Can you work these out from the model? Positions are in its coordinate system, mm. Face numbers are marked on the shaded views. A direction names the side the tool comes from. Coordinates: 2 decimals unless noted, no trailing zeros. Loops run counter-clockwise (first coordinate to the right, second up) from the corner with the lowest first, then second, coordinate; pieces in that order, holes last. Notation, with made-up numbers: (-36, 31) -> (18, 31) arc R7 ccw to (18, 35) -> close; hole circle Ø6 at (-19.5, 87). An arc over 180 degrees is marked (long way). Put each result on its own line as item: value. Start each with the question number.
Item 1: If we section it at A-A on x = 74: State how many separate pieces and enclosed holes the cut face has, plus the area to 3 significant figures.
Item 2: Will these pins go through, and if not, where does the flat tip stop? P1, Ø2.5, axis at y = 9, z = 7, coming from the +X side; P2, Ø2.5, axis at y = 40, z = 6.5, coming from the +X side; P3, Ø2, axis at y = 11.5, z = 1, coming from the -X side; P4, Ø1.5, axis at y = -5, z = 4.5, coming from the +X side.
Item 3: We'd pull the mould along Y, two halves only. Please class the marked faces 1, 2 and 3: pulls with the +Y half, pulls with the -Y half, needs draft (parallel to the pull), parting line crosses it, or undercut.
Item 4: Please list where these lines run through material, in increasing order: L1, parallel to Y at x = 74, z = 3.45; L2, parallel to Y at x = 74, z = 0.7; L3, parallel to X at y = -1, z = 3. Write a range as from..to.
Item 5: For the marked faces 4 and 5, which set-ups out of +Z, -Z, +X, -X, +Y, -Y let a thin tool reach every point of the face, with its end or its side?
Item 6: If we section it at C-C on x = 0: Please give me the cut outline in (y, z), plus the area to 3 significant figures.
```python
from build123d import *

# Parameters (mm, degrees)
SKETCH1_R           = 3.05
SKETCH1_R_2         = 1.55
BOSS_EXTRUDE1_DEPTH = 9
CUT_EXTRUDE1_DEPTH  = 5
CHAMFER2_SIZE       = 2.7
SKETCH3_W           = 38
SKETCH3_H           = 38
CUT_EXTRUDE2_DEPTH  = 96.66216598
FILLET1_R           = 4
CHAMFER3_SIZE       = 2
SKETCH4_R           = 3.35
CUT_EXTRUDE3_DEPTH  = 1
CHAMFER4_SIZE       = 1.8


with BuildPart() as part:
    # Sketch1 → Boss-Extrude1 (new body)
    with BuildSketch(Plane.XY):
        with BuildLine():
            Line((84, 45.5), (84, 24))
            Line((84, 24), (84, -14.5))
            Line((84, -14.5), (84, -26.5))
            Line((84, -26.5), (18, -26.5))
            Line((18, -26.5), (-9.05, -8.967177323))
            Line((-9.05, -8.967177323), (-9.05, 0))
            ThreePointArc((-9.05, 0), (-8.604128548, 2.805614358), (-7.310448193, 5.334777148))
            Line((-7.310448193, 5.334777148), (22, 45.5))
            Line((22, 45.5), (84, 45.5))
        make_face()
        with Locations((34, 35.5)):
            Circle(SKETCH1_R, mode=Mode.SUBTRACT)
        with Locations((54, 35.5)):
            Circle(SKETCH1_R, mode=Mode.SUBTRACT)
        with Locations((74, 35.5)):
            Circle(SKETCH1_R_2, mode=Mode.SUBTRACT)
        with Locations((74, -20.5)):
            Circle(SKETCH1_R_2, mode=Mode.SUBTRACT)
        with BuildLine():
            Line((43, 23.5), (43, 7.5))
            ThreePointArc((43, 7.5), (46, 4.5), (43, 1.5))
            Line((43, 1.5), (43, -16.5))
            Line((43, -16.5), (21.932011766, -16.5))
            Line((21.932011766, -16.5), (4.640610801, -3.881653178))
            ThreePointArc((4.640610801, -3.881653178), (-5.977483288, -0.933913025), (3.235425713, 5.112193312))
            Line((3.235425713, 5.112193312), (12.805005626, 18.22575293))
            ThreePointArc((12.805005626, 18.22575293), (14.884756486, 20.397148397), (13.451233091, 17.75417042))
            Line((13.451233091, 17.75417042), (3.881653178, 4.640610801))
            ThreePointArc((3.881653178, 4.640610801), (5.977483288, 0.933913025), (5.112193312, -3.235425713))
            Line((5.112193312, -3.235425713), (21.021073392, -14.84488216))
            ThreePointArc((21.021073392, -14.84488216), (23.110996656, -15.009801956), (24.2, -13.218419945))
            Line((24.2, -13.218419945), (24, 23.5))
            Line((24, 23.5), (43, 23.5))
        make_face(mode=Mode.SUBTRACT)
    extrude(amount=BOSS_EXTRUDE1_DEPTH)

    # Sketch2 → Cut-Extrude1 (cut)
    with BuildSketch(Plane.XY.offset(9)):
        Polygon((24, 25.5), (22, 25.5), (22, -12.5), (26, -16.5), (34, -16.5), (34, -26.5), (52, -26.5), (52, -16.5), (64, -16.5), (64, -26.5), (84, -26.5), (84, 45.5), (24, 45.5), align=None)
    extrude(amount=-CUT_EXTRUDE1_DEPTH, mode=Mode.SUBTRACT)

    # Chamfer2
    chamfer2_edges = [part.edges().sort_by_distance(p)[0] for p in [
        (30.95, 35.5, 0),
        (50.95, 35.5, 0),
    ]]
    chamfer(chamfer2_edges, length=CHAMFER2_SIZE)

    # Sketch3 → Cut-Extrude2 (cut, through all)
    with BuildSketch(Plane.XY.offset(4)):
        with Locations((43, 4.5)):
            Rectangle(SKETCH3_W, SKETCH3_H)
    extrude(amount=-CUT_EXTRUDE2_DEPTH, mode=Mode.SUBTRACT)

    # Fillet1
    fillet1_edges = [part.edges().sort_by_distance(p)[0] for p in [
        (62, 23.5, 2),
        (62, -14.5, 2),
        (24, 23.5, 2),
    ]]
    fillet(fillet1_edges, radius=FILLET1_R)

    # Chamfer3
    chamfer3_edges = [part.edges().sort_by_distance(p)[0] for p in [
        (22, 25.5, 6.5),
    ]]
    chamfer(chamfer3_edges, length=CHAMFER3_SIZE - 0.0001)  # a hair under: the kernel refuses the full size

    # Sketch4 → Cut-Extrude3 (cut)
    with BuildSketch(Plane(origin=(0, 0, 0), x_dir=(-1, 0, 0), z_dir=(0, 0, -1))):
        with Locations((-74, 35.5)):
            Circle(SKETCH4_R)
        with Locations((-74, -20.5)):
            Circle(SKETCH4_R)
    extrude(amount=-CUT_EXTRUDE3_DEPTH, mode=Mode.SUBTRACT)

    # Chamfer4
    chamfer4_edges = [part.edges().sort_by_distance(p)[0] for p in [
        (72.45, 35.5, 1),
        (72.45, -20.5, 1),
    ]]
    chamfer(chamfer4_edges, length=CHAMFER4_SIZE - 0.0001)  # a hair under: the kernel refuses the full size


solid = part.part
```
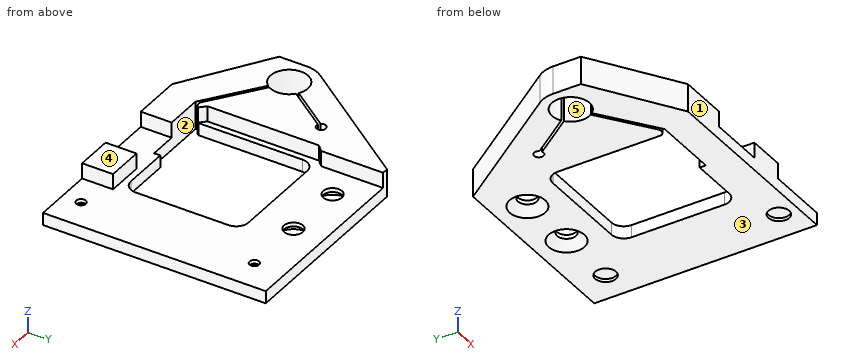
Solutions:
1. separate pieces: 3
1. enclosed holes: 0
1. area: 250 mm^2
2. P1: x = 22
2. P2: x = 24
2. P3: x = -3.54
2. P4: x = 84
3. face 1: pulls with the -Y half
3. face 2: undercut
3. face 3: needs draft
4. L1: -26.5..-22.05, -18.95..33.95, 37.05..45.5
4. L2: -26.5..-23.85, -17.15..32.15, 38.85..45.5
4. L3: -9.05..-5.97, 5.97..24, 62..84
5. face 4: +Z, +X, -X, +Y, -Y
5. face 5: +Z, -Z
6. outline: (-14.83, 0) -> (-6.05, 0) -> (-6.05, 9) -> (-14.83, 9) -> close; (6.05, 0) -> (15.35, 0) -> (15.35, 9) -> (6.05, 9) -> close
6. area: 163 mm^2
